Verification items for the finished model (mm, model axes). Coordinates: 2 decimals unless noted, no trailing zeros.
Q1. Thickness scan on line 1 (Z direction, x = 0, y = 1.4); line 2 (X direction, y = 1.05, z = 83.82); line 3 (Z direction, x = -28.5, y = 0.1). Record the ranges inside material, lowest first.
Q2. Draft check along X on faces 1 (the cylindrical face through (-0.806, 0.74, 82.555)), 2 (the flat face through (3, 1, 41)), 3 (the flat face through (-14, 1.5, 43)). Enter one of: pulls with the +X half, pulls with the -X half, needs draft (parallel to the pull), parting line crosses it, or undercut.
Q3. Depth check by flat-ended pin: P1, Ø2.5, axis at x = -29.141, z = 0, coming from the -Y side. Enter the tip coordinate at first touch or a pass-through.
Autodesk Inventor part; units mm, degrees
ref_plane "YZ Plane" through (0, 0, 0) normal (1, 0, 0) x (0, 1, 0)
ref_plane "XZ Plane" through (0, 0, 0) normal (0, 1, 0) x (-1, 0, 0)
ref_plane "XY Plane" through (0, 0, 0) normal (0, 0, 1) x (1, 0, 0)
sketch "Sketch1" plane through (0, 0, 0) normal (0, 1, 0) x (-1, 0, 0)
  line L0 (0, 0) -> (29.141, 0)
  line L1 (29.141, 83.82) -> (0, 83.82)
  line L2 (0, 83.82) -> (0, 86.82)
  line L3 (0, 86.82) -> (-3, 86.82)
  line L4 (-3, 86.82) -> (32.141, 86.82)
  line L5 (32.141, 86.82) -> (32.141, -3)
  line L6 (32.141, -3) -> (-3, -3)
  line L7 (-3, -3) -> (-3, 86.82)
  circle A0 centre (0, 83.82) radius 1.5
  circle A1 centre (29.141, 83.82) radius 1.5
  circle A2 centre (0, 0) radius 1.5
  circle A3 centre (29.141, 0) radius 1.5
  dimension "d0" = 29.141
  dimension "d1" = 83.82
  dimension "d2" = 3
  dimension "d3" = 3
  dimension "d4" = 35.141
  dimension "d5" = 89.82
  dimension "d6" = 3
  dimension "d7" = 3
  dimension "d8" = 3
  dimension "d9" = 3
extrude "Extrusion1" add sketch "Sketch1" along normal blind 1.5
fillet "Fillet1" radius 3 4 edges at (-32.141, 0.75, 86.82) (3, 0.75, 86.82) (3, 0.75, -3) (-32.141, 0.75, -3)
properties part number "Power Supply"
Check values:
1. line 1: z = -3 to -1.5, 1.5 to 82.32, 85.32 to 86.82
1. line 2: x = -32.14 to -30.64, -27.64 to -1.5, 1.5 to 3
1. line 3: z = -3 to -1.36, 1.36 to 82.46, 85.18 to 86.82
2. face 1: undercut
2. face 2: pulls with the +X half
2. face 3: needs draft
3. P1: passes through
